from build123d import *

# Parameters (mm, degrees)
F0_W     = 3.75
F0_H     = 11
F1_DEPTH = 24
F3_DEPTH = 24.001
F4_D     = 4.6
F5_R     = 1.99999
F6_R     = 5


# Not quite as in the source:
# - a fillet or chamfer is up to 0.001 mm smaller than in the source, because OpenCascade refuses the exact size


with BuildPart() as f1:
    # F0 (on Front) → F1 (new body)
    with BuildSketch(Plane.XZ):
        Polygon((0, 0), (-4.25, 0), (-8, 0), (-28, 0), (-28, -12), (-12, -12), (-12, -16), (-28, -16), (-28, -28), (0, -28), (0, -24), (-8, -24), (-24, -24), (-24, -20), (-8, -20), (-8, -11), (-8, -8), (-24, -8), (-24, -4), (-8, -4), (0, -4), align=None)
        Polygon((28, 0), (8, 0), (8, -4), (24, -4), (24, -8), (8, -8), (8, -11), (8, -20), (24, -20), (24, -24), (8, -24), (0, -24), (0, -28), (28, -28), (28, -16), (12, -16), (12, -12), (28, -12), align=None)
        Polygon((8, -4), (8, 0), (4.25, 0), (0, 0), (0, -4), align=None)
        with Locations((6.125, 5.5)):
            Rectangle(F0_W, F0_H)
        Polygon((4.25, 0), (4.25, 11), (-4.25, 11), (-4.25, 0), (0, 0), align=None)
        with Locations((-6.125, 5.5)):
            Rectangle(F0_W, F0_H)
    extrude(amount=F1_DEPTH)

    # F0 (on Front) → F3 (cut, through all)
    with BuildSketch(Plane.XZ):
        Polygon((4.25, 0), (4.25, 11), (-4.25, 11), (-4.25, 0), (0, 0), align=None)
    extrude(amount=F3_DEPTH, mode=Mode.SUBTRACT)

    # F4 (through all)
    with Locations(Plane.YZ.offset(8)):
        with Locations((-10, 6)):
            Hole(F4_D / 2)

    # F5 (radius 2 in the source; OpenCascade refuses exactly that, so slightly less here)
    f5_edges = [f1.edges().sort_by_distance(p)[0] for p in [
        (12, -12, -16),
        (-24, -12, -24),
        (-24, -12, -8),
        (12, -12, -12),
        (24, -12, -8),
        (24, -12, -24),
        (-12, -12, -12),
        (24, -12, -20),
        (24, -12, -4),
        (-24, -12, -20),
        (-24, -12, -4),
        (-12, -12, -16),
        (-8, -12, 11),
        (-6.125, -24, 11),
        (6.125, -24, 11),
        (8, -12, 11),
        (-8, 0, 5.5),
        (-8, -24, 5.5),
        (-6.125, 0, 11),
        (6.125, 0, 11),
        (8, 0, 5.5),
        (8, -24, 5.5),
    ]]
    fillet(f5_edges, radius=F5_R)

    # F6
    f6_edges = [f1.edges().sort_by_distance(p)[0] for p in [
        (-28, -12, -28),
        (-28, -12, -16),
        (-28, -12, -12),
        (-28, -12, 0),
        (8, -12, -8),
        (8, -12, -20),
        (-8, -12, -8),
        (-8, -12, -20),
        (28, -12, 0),
        (28, -12, -12),
        (28, -12, -16),
        (28, -12, -28),
    ]]
    fillet(f6_edges, radius=F6_R)


solid = f1.part
Can you work these out from the model? Positions are in its coordinate system, mm. A direction names the side the tool comes from. Coordinates: 2 decimals unless noted, no trailing zeros. Loops run counter-clockwise (first coordinate to the right, second up) from the corner with the lowest first, then second, coordinate; pieces in that order, holes last. Notation, with made-up numbers: (47, 2) - (82, 2) arc R10 cw to (82, 9) - close; hole circle Ø7 at (-5, 30.25). An arc over 180 degrees is marked (long way). Put each result on its own line as item: value. Start each with the question number.
Item 1: Which directions (+Z, -Z, +X, -X, +Y, -Y) give clear straight access to the entire face, cutting with the end or side of a thin tool? Please do faces 5 (the face through (-4.25, -12, 4)), 6 (the face through (-12.6, -12.17, -15.43)), 7 (the face through (28, -12, -6)), 8 (the face through (26, -12, -17)), 9 (the face through (-18, -12, -20)).
Item 2: Suppose I cut it at B-B (x = -9). Please give me the cut outline in (y, z).
Item 3: If we mould it in two halves opening along X, with no side actions, what happens to faces 1 (the face through (23.43, -12.17, -7.4)), 2 (the face through (-28, -12, -22)), 3 (the face through (23.4, -12.17, -20.57)), 4 (the face through (0, 0, -1))? For each: +X half, -X half, draft (parallel to the pull), parting line (faces both ways), or undercut.
Item 4: If I drill on line 1 along Z through (x, y) = (5.4, -10); line 2 along Z through (x, y) = (-22.5, -8); line 3 along X through (y, z) = (-4, 8), over which ranges is the centre line in solid material (lowest first)?
Item 5: For pin 1 (2 mm diameter, centred on y = -13, z = -14, fed in from -X); pin 2 (5.5 mm diameter, centred on y = -17, z = 4.5, fed in from +X); pin 3 (5 mm diameter, centred on x = 17, y = -19, fed in from +Z), each with a flat end and sliding along its axis, tell me the tip position at first contact or that it passes through.
Item 6: Suppose I cut it at C-C (y = -10). State how many separate pieces and enclosed holes the cut face has, and give its area (3 significant figures).
Item 7: Suppose I cut it at A-A (z = 6). Please give me the cut outline in (x, y).
Here are the results:
1. face 5: +Z, +Y, -Y
1. face 6: -X, +Y, -Y
1. face 7: +Z, -Z, +X, +Y, -Y
1. face 8: +X, +Y, -Y
1. face 9: +Y, -Y
2. outline: (-24, -28) - (0, -28) - (0, -24) - (-24, -24) - close; (-24, -18) - (0, -18) - (0, -10) - (-24, -10) - close; (-24, -4) - (0, -4) - (0, 0) - (-24, 0) - close
3. face 1: undercut
3. face 2: -X half
3. face 3: undercut
3. face 4: draft
4. line 1: -28 to -24, -4 to 3.7, 8.3 to 11
4. line 2: -28 to -23.94, -20.06 to -16, -12 to -7.94, -4.06 to 0
4. line 3: -8 to -4.25, 4.25 to 8
5. pin 1: x = -12.27
5. pin 2: x = 8
5. pin 3: z = 0
6. separate pieces: 3
6. enclosed holes: 1
6. area: 856 mm²
7. outline: (-8, -22) arc R2 ccw to (-6, -24) - (-4.25, -24) - (-4.25, -12.3) - (-8, -12.3) - close; (-8, -7.7) - (-4.25, -7.7) - (-4.25, 0) - (-6, 0) arc R2 ccw to (-8, -2) - close; (4.25, -24) - (6, -24) arc R2 ccw to (8, -22) - (8, -12.3) - (4.25, -12.3) - close; (4.25, -7.7) - (8, -7.7) - (8, -2) arc R2 ccw to (6, 0) - (4.25, 0) - close
